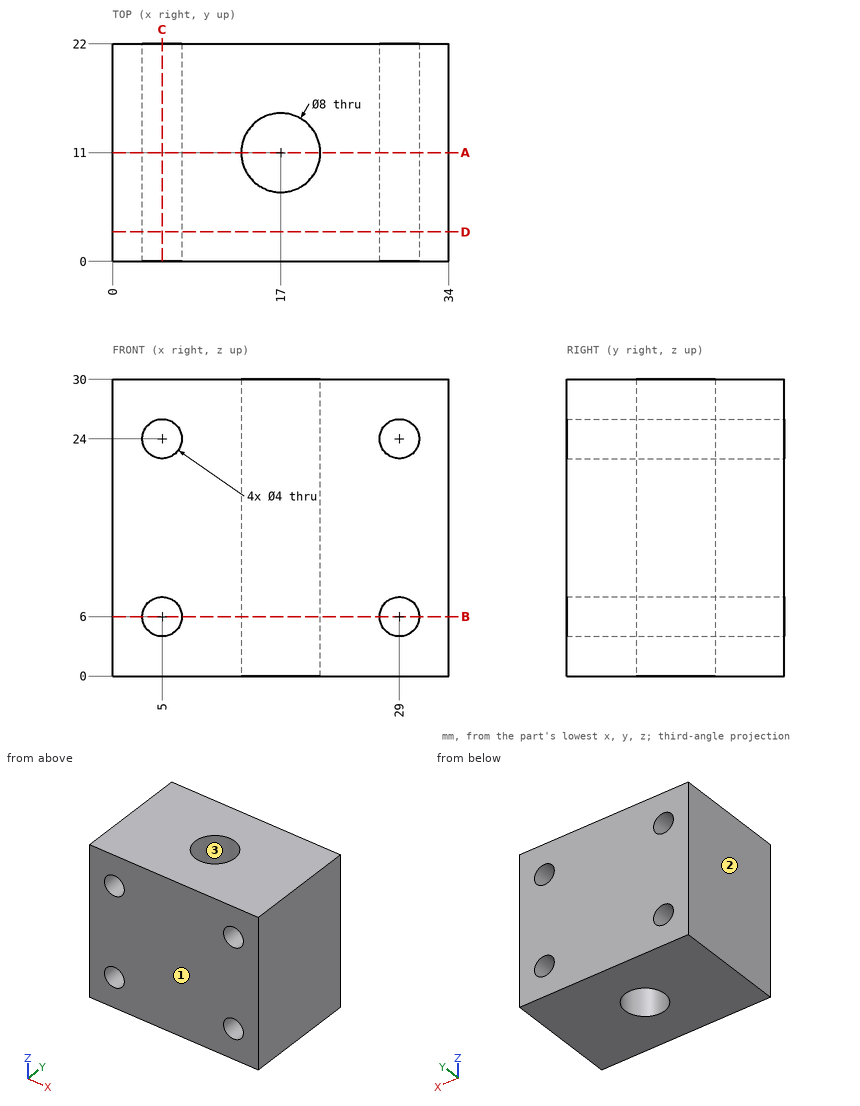
The drawing under review shows one solid part. Ordinate dimensions are in mm from its lowest x, y, z. Give positions to 0.01 mm unless a question says otherwise; leave off trailing zeros. Order: outer loops, then holes, each group sorted by start corner. A loop starts at its lowest first (then second) coordinate and runs counter-clockwise, first axis right, second up. Notation, with made-up numbers: M 3.25,63 L 9.25,63 A22 cw 9.25,94 Z; hole C -6.5,38.5 d9. An arc over 180 degrees is marked long. One line per question, with ' | ' between items. Start each with the question number.
Q1. We need section A-A (y = 11). Write out the cut boundary in (x, z).
Q2. We need section B-B (z = 6). Write out the cut boundary in (x, y).
Q3. For L1, parallel to Z at x = 5, y = 7.5; L2, parallel to Y at x = 17, z = 14.25; L3, parallel to X at y = 6, z = 6, list the stretches that pass through material, from the lowest coordinate up. Write a range as [from, to].
Q4. We need section D-D (y = 3). Write out the cut boundary in (x, z), plus the area to 3 significant figures.
Q5. We need section C-C (x = 5). Write out the cut boundary in (y, z), plus the area to 3 significant figures.
Q6. The part is to be moulded in two halves that separate along X. For the marked faces 1, 2 and 3, say which applies: +X half, -X half, draft (parallel to the pull), parting line (faces both ways), or undercut.
Q7. For pin 1 Ø3.5 at (x, z) = (5, 6) entering from +Y, flat-tipped, find the tip position at first contact; note if it passes through.
Returned:
1) outline: M 0,0 L 13,0 L 13,30 L 0,30 Z; M 21,0 L 34,0 L 34,30 L 21,30 Z; hole C 5,6 d4; hole C 5,24 d4; hole C 29,6 d4; hole C 29,24 d4
2) outline: M 0,0 L 3,0 L 3,22 L 0,22 Z; M 7,0 L 27,0 L 27,22 L 7,22 Z; M 31,0 L 34,0 L 34,22 L 31,22 Z; hole C 17,11 d8
3) L1: [0, 4], [8, 22], [26, 30] | L2: [0, 7], [15, 22] | L3: [0, 3], [7, 27], [31, 34]
4) outline: M 0,0 L 34,0 L 34,30 L 0,30 Z; hole C 5,6 d4; hole C 5,24 d4; hole C 29,6 d4; hole C 29,24 d4 | area: 970 mm2
5) outline: M 0,0 L 22,0 L 22,4 L 0,4 Z; M 0,8 L 22,8 L 22,22 L 0,22 Z; M 0,26 L 22,26 L 22,30 L 0,30 Z | area: 484 mm2
6) face 1: draft | face 2: -X half | face 3: undercut
7) pin 1: through
